```python
from build123d import *

# Parameters (mm, degrees)
SKETCH_R          = 27.5
SKETCH_R_2        = 19.5
PAD_DEPTH         = 10
SKETCH001_R       = 1.5
POCKET_DEPTH      = 10
SKETCH002_R       = 1.5
POCKET001_DEPTH   = 1.5
COPYSKETCH003_R   = 23.5
COPYSKETCH003_R_2 = 19.5
POCKET002_DEPTH   = 5


with BuildPart() as part:
    # Sketch → Pad (new body)
    with BuildSketch(Plane.XY):
        Circle(SKETCH_R)
        Circle(SKETCH_R_2, mode=Mode.SUBTRACT)
    extrude(amount=PAD_DEPTH)

    # Sketch001 → Pocket (cut)
    with BuildSketch(Plane(origin=(27.5, 0, 0), x_dir=(1, 0, 0), z_dir=(0, 0, 1))):
        Circle(SKETCH001_R)
    extrude(amount=POCKET_DEPTH, mode=Mode.SUBTRACT)

    # Sketch002 → Pocket001 (cut)
    with BuildSketch(Plane.YZ.offset(27.5)):
        Circle(SKETCH002_R)
    extrude(amount=-POCKET001_DEPTH, mode=Mode.SUBTRACT)

    # CopySketch003 → Pocket002 (cut)
    with BuildSketch(Plane.XY.offset(5)):
        Circle(COPYSKETCH003_R)
        Circle(COPYSKETCH003_R_2, mode=Mode.SUBTRACT)
    extrude(amount=POCKET002_DEPTH, mode=Mode.SUBTRACT)


solid = part.part
```
The listing builds one solid part. Answer for the finished solid, in the listing's coordinates (mm). A direction names the side the tool comes from. Give positions to 0.01 mm unless a question says otherwise; leave off trailing zeros. Write each loop counter-clockwise with the first axis right and the second up, starting at its lowest first coordinate (ties: lowest second). Pieces come first, ordered by that corner, then holes. Notation, with made-up numbers: (35, -10) -> (91, -10) arc R18 cw to (91, 12) -> close; hole circle Ø2 at (-32, 62). An arc over 180 degrees is marked (long way). Use one line per item in the form item = value.
1) Each of these flat-tipped pins is pushed along its axis until it touches: P1, Ø1.5, axis at y = -20.5, z = 6, coming from the -X side; P2, Ø2, axis at x = 15, z = 1.5, coming from the -Y side; P3, Ø6, axis at x = 2.5, z = 6, coming from the +Y side. Where does it stop, or does it pass through?
Result:
P1 = -19.14
P2 = -23.67
P3 = 27.5
2) A tool of negligible diameter and unlimited length cuts with its end or side. For faces 1 (the cylindrical face through (22.4, 7.1, 7.5)), 2 (the cylindrical face through (26, 0, 5)), 3 (the flat face through (26, 0, 1)), from which of +Z, -Z, +X, -X, +Y, -Y can it reach the whole face along a straight path? Write none if from no direction.
Result:
face_1 = +Z
face_2 = +Z, -Z, +X
face_3 = -Z, +X
3) Straight lines are drawn through the part: probe 1 along Y at (x, z) = (0, 7.2); probe 2 along Y at (x, z) = (0, 3.3); probe 3 along Z at (x, y) = (9.5, 21). For each, find the intervals that lie inside material, in ascending order.
Result:
probe_1 = -27.5 to -23.5, 23.5 to 27.5
probe_2 = -27.5 to -19.5, 19.5 to 27.5
probe_3 = 0 to 5
4) Section C-C on z = 4 is taken. Write down the section's boundary in (x, y).
Result:
outline = (27.46, -1.5) arc R1.5 cw to (27.46, 1.5) arc R27.5 ccw (long way) to start; hole circle Ø39 at (0, 0)
5) Section A-A on x = 0 is taken. Write down the section's boundary in (y, z), plus the area to 3 significant figures.
Result:
outline = (-27.5, 0) -> (-19.5, 0) -> (-19.5, 5) -> (-23.5, 5) -> (-23.5, 10) -> (-27.5, 10) -> close; (19.5, 0) -> (27.5, 0) -> (27.5, 10) -> (23.5, 10) -> (23.5, 5) -> (19.5, 5) -> close
area = 120 mm²
6) Section B-B on y = -13 is taken. Write down the section's boundary in (x, z).
Result:
outline = (-24.23, 0) -> (-14.53, 0) -> (-14.53, 5) -> (-19.58, 5) -> (-19.58, 10) -> (-24.23, 10) -> close; (14.53, 0) -> (24.23, 0) -> (24.23, 10) -> (19.58, 10) -> (19.58, 5) -> (14.53, 5) -> close
